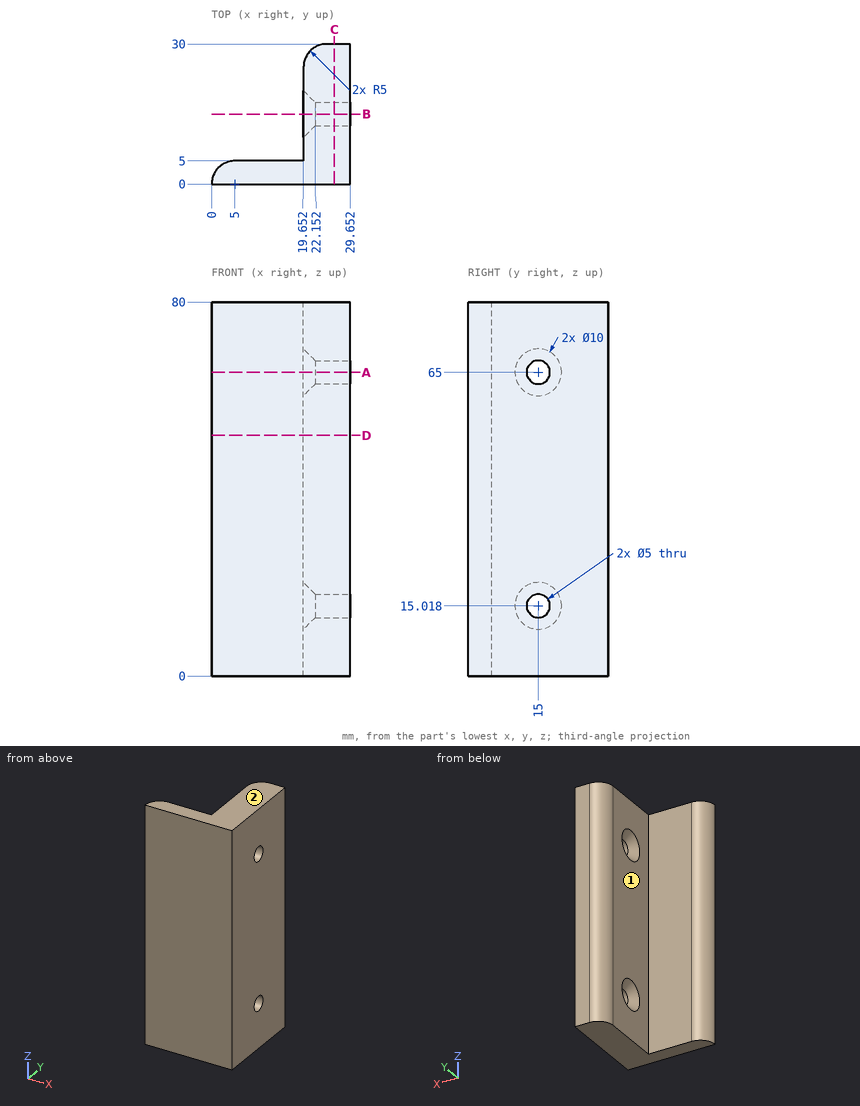
Input: dimensioned drawing with shaded views. Units: mm. Origin: part minimum x, y, z. A direction names the side the tool comes from. Round coordinates to 2 decimals unless told otherwise and drop trailing zeros. Loops run counter-clockwise (first coordinate to the right, second up) from the corner with the lowest first, then second, coordinate; pieces in that order, holes last. Notation, with made-up numbers: (17.5, 19) -> (30.5, 19) arc R8 ccw to (30.5, 31) -> close; hole circle Ø10 at (-36.5, 43.25). An arc over 180 degrees is marked (long way). Use one line per item in the form item = value. Start each with the question number.
1) Line query: L1, parallel to Z at x = 26, y = 15; L2, parallel to Y at x = 7, z = 10; L3, parallel to Y at x = 28, z = 65. Output: solid intervals per line, ascending.
2) Section B-B on y = 15. Output: boundary loops of the cut face in (x, z).
3) First-contact query: P1, Ø4, axis at x = 19.5, y = 9, coming from the -Z side; P2, Ø16, axis at x = 10.5, z = 25.5, coming from the +Y side. Flat tips, straight axial feed; report the tip coordinate or a pass-through.
4) Section A-A on z = 65. Output: boundary loops of the cut face in (x, y), then the cut area to 3 significant figures.
5) Section C-C on x = 26.25. Output: boundary loops of the cut face in (y, z).
6) Access query for the marked faces 1 and 2. Directions: +Z, -Z, +X, -X, +Y, -Y. A direction counts if a zero-diameter tool reaches every point of the face in a straight line with its end or side. Return the directions, or none.
7) Section D-D on z = 51.5. Output: boundary loops of the cut face in (x, y).
Response:
q1.L1 = 0 to 12.52, 17.52 to 62.5, 67.5 to 80
q1.L2 = 0 to 5
q1.L3 = 0 to 12.5, 17.5 to 30
q2.outline = (19.65, 0) -> (29.65, 0) -> (29.65, 12.52) -> (22.15, 12.52) -> (19.65, 10.02) -> close; (19.65, 20.02) -> (22.15, 17.52) -> (29.65, 17.52) -> (29.65, 62.5) -> (22.15, 62.5) -> (19.65, 60) -> close; (19.65, 70) -> (22.15, 67.5) -> (29.65, 67.5) -> (29.65, 80) -> (19.65, 80) -> close
q3.P1 = 0
q3.P2 = 5
q4.outline = (0, 0) -> (29.65, 0) -> (29.65, 12.5) -> (22.15, 12.5) -> (19.65, 10) -> (19.65, 5) -> (5, 5) arc R5 ccw to start; (19.65, 20) -> (22.15, 17.5) -> (29.65, 17.5) -> (29.65, 30) -> (24.65, 30) arc R5 ccw to (19.65, 25) -> close
q4.area = 331 mm^2
q5.outline = (0, 0) -> (30, 0) -> (30, 80) -> (0, 80) -> close; hole circle Ø5 at (15, 15.02); hole circle Ø5 at (15, 65)
q6.face_1 = +Z, -Z, -X, +Y
q6.face_2 = +Z, +X, -X, +Y, -Y
q7.outline = (0, 0) -> (29.65, 0) -> (29.65, 30) -> (24.65, 30) arc R5 ccw to (19.65, 25) -> (19.65, 5) -> (5, 5) arc R5 ccw to start
